```python
from build123d import *

# Parameters (mm, degrees)
F0_R     = 17.5
F1_DEPTH = 20


with BuildPart() as f1:
    # F0 (on Front) → F1 (new body)
    with BuildSketch(Plane.XZ):
        with BuildLine():
            Line((45, 0), (20, 0))
            ThreePointArc((20, 0), (0, 20), (-20, 0))
            Line((-20, 0), (-45, 0))
            Line((-45, 0), (-45, -2.778499))
            Line((-45, -2.778499), (-19.797258, -2.840526))
            ThreePointArc((-19.797258, -2.840526), (-0.049222, -19.999939), (19.783036, -2.937938))
            Line((19.783036, -2.937938), (45, -3))
            Line((45, -3), (45, 0))
        make_face()
        Circle(F0_R, mode=Mode.SUBTRACT)
    extrude(amount=F1_DEPTH)


solid = f1.part
```
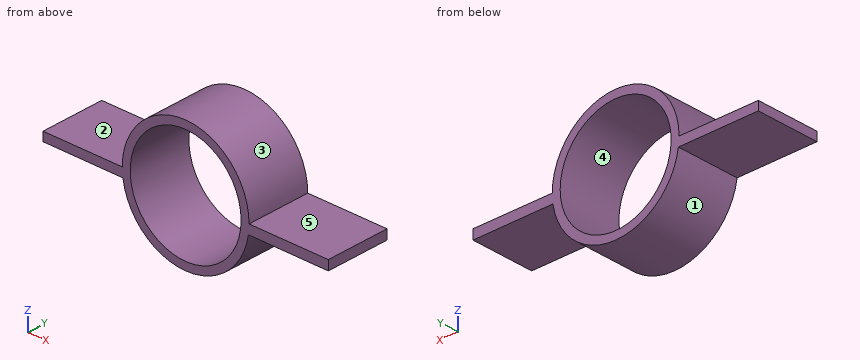
CAD build for the part. Positions are in the model's coordinates, mm. Face numbers are marked on the shaded views. A direction names the side the tool comes from. Round coordinates to 2 decimals unless told otherwise and drop trailing zeros. Write each loop counter-clockwise with the first axis right and the second up, starting at its lowest first coordinate (ties: lowest second). Pieces come first, ordered by that corner, then holes. Notation, with made-up numbers: (33.25, 18.25) - (77.25, 18.25) arc R32 cw to (77.25, 55.25) - close; hole circle Ø11 at (-36, -4.5). An arc over 180 degrees is marked (long way). Write item = value, one per line. Start each with the question number.
Q1. Band-saw the part on B-B (y = -10). Give the cut face in (x, z).
Q2. Drop flat-ended pins along their axis: pin 1 (6 mm diameter, centred on y = -5, z = 13, fed in from -X); pin 2 (3 mm diameter, centred on x = -9.5, y = -14, fed in from +Z); pin 3 (6 mm diameter, centred on x = 27, y = -7, fed in from +Z); pin 4 (6 mm diameter, centred on x = -13, z = 1, fed in from +Y). Give the stop position or say it passes through.
Q3. Probe L1, parallel to Z at x = 0, y = -13.25; L2, parallel to Z at x = 11.5, y = -8.25; L3, parallel to X at y = -6, z = -10. List the from-to ranges inside material, lowest first. Write a range as from..to.
Q4. Band-saw the part on A-A (x = 0). Give the cut face in (y, z), then the cut area to 4 significant figures.
Q5. Mould opens along X. For the marked faces 3, 4 and 5 say: pulls with the +X half, pulls with the -X half, needs draft (parallel to the pull), parting line crosses it, or undercut.
Q6. Band-saw the part on D-D (x = -39). Give the cut face in (y, z), then the cut area to 3 significant figures.
Q7. Which spindle directions (+Z, -Z, +X, -X, +Y, -Y) get a long thin tool onto all of the face, cutting with end or side? Do the marked faces 1 and 2. Say none if no direction does.
Q8. Band-saw the part on C-C (z = 7). Give the cut face in (x, y) (3 decimals), then the cut area to 3 significant figures.
Answers below:
q1.outline = (-45, -2.78) - (-19.8, -2.84) arc R20 ccw to (19.78, -2.94) - (45, -3) - (45, 0) - (20, 0) arc R20 ccw to (-20, 0) - (-45, 0) - close; hole circle Ø35 at (0, 0)
q2.pin_1 = -17.32
q2.pin_2 = 18.33
q2.pin_3 = 0
q2.pin_4 = through
q3.L1 = -20..-17.5, 17.5..20
q3.L2 = -16.36..-13.19, 13.19..16.36
q3.L3 = -17.32..-14.36, 14.36..17.32
q4.outline = (-20, -20) - (0, -20) - (0, -17.5) - (-20, -17.5) - close; (-20, 17.5) - (0, 17.5) - (0, 20) - (-20, 20) - close
q4.area = 100.0 mm2
q5.face_3 = parting line crosses it
q5.face_4 = undercut
q5.face_5 = needs draft
q6.outline = (-20, -2.79) - (0, -2.79) - (0, 0) - (-20, 0) - close
q6.area = 55.9 mm2
q7.face_1 = -Z, +Y, -Y
q7.face_2 = +Z, -X, +Y, -Y
q8.outline = (-18.735, -20) - (-16.039, -20) - (-16.039, 0) - (-18.735, 0) - close; (16.039, -20) - (18.735, -20) - (18.735, 0) - (16.039, 0) - close
q8.area = 108 mm2
